```python
from build123d import *

# Parameters (mm, degrees)
SKETCH_W             = 130
SKETCH_H             = 240
PAD_DEPTH            = 10
SKETCH015_R          = 1.75
POCKET008_DEPTH      = 10.001
POCKET008_DEPTH_BACK = 0.001
SKETCH016_R          = 4
POCKET009_DEPTH      = 3


with BuildPart() as part:
    # Sketch → Pad (new body)
    with BuildSketch(Plane.XY):
        Rectangle(SKETCH_W, SKETCH_H)
    extrude(amount=PAD_DEPTH)

    # Sketch015 (on Face6 of Pad) → Pocket008 (cut, two sides)
    with BuildSketch(Plane.XY.offset(10)) as pocket008_sk:
        with Locations((47, 68.5)):
            Circle(SKETCH015_R)
        with Locations((21, 19.5)):
            Circle(SKETCH015_R)
        with Locations((-12, 19.5)):
            Circle(SKETCH015_R)
        with Locations((-37, -54)):
            Circle(SKETCH015_R)
    extrude(amount=-POCKET008_DEPTH, mode=Mode.SUBTRACT)
    extrude(pocket008_sk.sketch, amount=POCKET008_DEPTH_BACK, mode=Mode.SUBTRACT)

    # Sketch016 (on Face4 of Pocket008) → Pocket009 (cut)
    with BuildSketch(Plane(origin=(0, 0, 0), x_dir=(1, 0, 0), z_dir=(0, 0, -1))):
        with Locations((-37, 54)):
            Circle(SKETCH016_R)
        with Locations((-12, -19.5)):
            Circle(SKETCH016_R)
        with Locations((21, -19.5)):
            Circle(SKETCH016_R)
        with Locations((47, -68.5)):
            Circle(SKETCH016_R)
    extrude(amount=-POCKET009_DEPTH, mode=Mode.SUBTRACT)


solid = part.part
```
Could you check a few things on this model? Use its own coordinates, in mm. A direction names the side the tool comes from. Round coordinates to 2 decimals unless told otherwise and drop trailing zeros. Answer in a Markdown table with one row per item. Add a question column.
Q1. On a 3-axis mill with a long thin cutter (end or side, diameter ignored), from which of +Z, -Z, +X, -X, +Y, -Y can I reach the whole of each face in a straight line? I mean faces 1 (the flat face through (-36, -52, 3)), 2 (the flat face through (-1, -120, 5)). Say none if no direction works.
Q2. Will these pins go through, and if not, where does the flat tip stop? pin 1 Ø4 at (x, y) = (-12, 21) entering from -Z; pin 2 Ø2 at (x, y) = (21, 19.5) entering from +Z.
Q3. If I drill on line 1 (X direction, y = 19.5, z = 2.3); line 2 (Y direction, x = 21, z = 5.5); line 3 (X direction, y = 68.5, z = 8.25), over which ranges is the centre line in solid material (lowest first)? Write a range as from..to.
Q4. If we mould it in two halves opening along X, with no side actions, what happens to faces 3 (the cylindrical face through (18.05, 16.8, 1.48)), 4 (the flat face through (-65, -2, 5)), 5 (the flat face through (65, -2, 5)), 6 (the flat face through (23, 20, 3))? For each: +X half, -X half, draft (parallel to the pull), parting line (faces both ways), or undercut.
Values:
| question | item | result |
|---|---|---|
| 1 | face 1 | -Z |
| 1 | face 2 | +Z, -Z, +X, -X, -Y |
| 2 | pin 1 | z = 3 |
| 2 | pin 2 | through |
| 3 | line 1 | -65..-16, -8..17, 25..65 |
| 3 | line 2 | -120..17.75, 21.25..120 |
| 3 | line 3 | -65..45.25, 48.75..65 |
| 4 | face 3 | undercut |
| 4 | face 4 | -X half |
| 4 | face 5 | +X half |
| 4 | face 6 | undercut |
